from build123d import *

# Parameters (mm, degrees)
SKETCH1_R           = 10
SKETCH1_R_2         = 1.65
BOSS_EXTRUDE1_DEPTH = 2
SKETCH2_R           = 16
BOSS_EXTRUDE2_DEPTH = 8
BOSS_EXTRUDE3_DEPTH = 12
SKETCH4_R           = 1.65
CUT_EXTRUDE1_DEPTH  = 12
SKETCH5_R           = 2.8
CUT_EXTRUDE2_DEPTH  = 5.6


with BuildPart() as part:
    # Sketch1 → Boss-Extrude1 (new body)
    with BuildSketch(Plane.XY):
        Circle(SKETCH1_R)
        with Locations((0, 7)):
            Circle(SKETCH1_R_2, mode=Mode.SUBTRACT)
        with Locations((7, 0)):
            Circle(SKETCH1_R_2, mode=Mode.SUBTRACT)
        with Locations((0, -7)):
            Circle(SKETCH1_R_2, mode=Mode.SUBTRACT)
        with Locations((-7, 0)):
            Circle(SKETCH1_R_2, mode=Mode.SUBTRACT)
    extrude(amount=BOSS_EXTRUDE1_DEPTH)

    # Sketch2 → Boss-Extrude2 (add)
    with BuildSketch(Plane.XY.offset(2)):
        Circle(SKETCH2_R)
    extrude(amount=BOSS_EXTRUDE2_DEPTH)

    # Sketch3 → Boss-Extrude3 (add)
    with BuildSketch(Plane.XY.offset(10)):
        Polygon((3.868246804, 0), (1.934123402, 3.35), (-1.934123402, 3.35), (-3.868246804, 0), (-1.934123402, -3.35), (1.934123402, -3.35), align=None)
    extrude(amount=BOSS_EXTRUDE3_DEPTH)

    # Sketch4 → Cut-Extrude1 (cut)
    with BuildSketch(Plane(origin=(0, 0, 0), x_dir=(-1, 0, 0), z_dir=(0, 0, -1))):
        with Locations(Location((0, -7, 0), (0, 0, 180))):
            Circle(SKETCH4_R)
        with Locations(Location((-7, 0, 0), (0, 0, 180))):
            Circle(SKETCH4_R)
        with Locations(Location((7, 0, 0), (0, 0, 180))):
            Circle(SKETCH4_R)
        with Locations(Location((0, 7, 0), (0, 0, 180))):
            Circle(SKETCH4_R)
    extrude(amount=-CUT_EXTRUDE1_DEPTH, mode=Mode.SUBTRACT)

    # Sketch5 → Cut-Extrude2 (cut)
    with BuildSketch(Plane.XY.offset(10)):
        with Locations((0, 7)):
            Circle(SKETCH5_R)
        with Locations((7, 0)):
            Circle(SKETCH5_R)
        with Locations((0, -7)):
            Circle(SKETCH5_R)
        with Locations((-7, 0)):
            Circle(SKETCH5_R)
    extrude(amount=-CUT_EXTRUDE2_DEPTH, mode=Mode.SUBTRACT)


solid = part.part
Check sheet for the modelled part. Datum: model origin and axes. Units: mm. A direction names the side the tool comes from. Round coordinates to 2 decimals unless told otherwise and drop trailing zeros. Write each loop counter-clockwise with the first axis right and the second up, starting at its lowest first coordinate (ties: lowest second). Pieces come first, ordered by that corner, then holes. Notation, with made-up numbers: (30.5, 16) - (78.5, 16) arc R20 ccw to (78.5, 49) - close; hole circle Ø2 at (84, -5.5). An arc over 180 degrees is marked (long way). Return JSON: item names as keys, results as strings.
Q1. Cross-section at D-D (z = 6). Record the boundary of the cut face in (x, y).
Returned:
{"outline": "circle Ø32 at (0, 0); hole circle Ø5.6 at (-7, 0); hole circle Ø5.6 at (0, -7); hole circle Ø5.6 at (0, 7); hole circle Ø5.6 at (7, 0)"}
Q2. Cross-section at B-B (y = -6). Record the boundary of the cut face in (x, z).
Returned:
{"outline": "(-14.83, 2) - (-8, 2) - (-8, 0) - (-1.31, 0) - (-1.31, 4.4) - (-2.62, 4.4) - (-2.62, 10) - (-14.83, 10) - close; (1.31, 0) - (8, 0) - (8, 2) - (14.83, 2) - (14.83, 10) - (2.62, 10) - (2.62, 4.4) - (1.31, 4.4) - close"}
Q3. Scan lines: L1, parallel to Y at x = 0, z = 2.1; L2, parallel to Y at x = 0, z = 8; L3, parallel to X at y = 2.5, z = 9.5. Record each from-to range of solid material in increasing order. Write a range as from..to.
Returned:
{"L1": "y = -16..-8.65, -5.35..5.35, 8.65..16", "L2": "y = -16..-9.8, -4.2..4.2, 9.8..16", "L3": "x = -15.8..-8.26, -5.74..5.74, 8.26..15.8"}
Q4. Access from +Z, -Z, +X, -X, +Y, -Y to the whole of each face (thin tool, end or side, straight path). Record for faces 4 (the cylindrical face through (-2.17, -9.76, 0.99)), 5 (the flat face through (0, 3.35, 16)), 6 (the cylindrical face through (-0.607, -9.733, 7.239)), 7 (the flat face through (-2.915, -1.652, 15.916)), 8 (the flat face through (2.888, -1.698, 15.916)).
Returned:
{"face 4": "-Z", "face 5": "+Z, +X, -X, +Y", "face 6": "+Z", "face 7": "+Z, -X, -Y", "face 8": "+Z, +X, -Y"}
Q5. Depth check by flat-ended pin: P1, Ø5, axis at x = 0.5, z = 17, coming from the +Y side; P2, Ø2, axis at x = -7, y = 9, coming from the -Z side; P3, Ø6, axis at x = -11, z = 9, coming from the -Y side. Enter the tip coordinate at first touch or a pass-through.
Returned:
{"P1": "stops at y = 3.35", "P2": "stops at z = 2", "P3": "stops at y = -13.86"}
Q6. Cross-section at C-C (x = -7). Record the boundary of the cut face in (y, z).
Returned:
{"outline": "(-14.39, 2) - (-7.14, 2) - (-7.14, 0) - (-1.65, 0) - (-1.65, 4.4) - (-2.8, 4.4) - (-2.8, 10) - (-14.39, 10) - close; (1.65, 0) - (7.14, 0) - (7.14, 2) - (14.39, 2) - (14.39, 10) - (2.8, 10) - (2.8, 4.4) - (1.65, 4.4) - close"}
Q7. Cross-section at A-A (x = 0). Record the boundary of the cut face in (y, z).
Returned:
{"outline": "(-16, 2) - (-10, 2) - (-10, 0) - (-8.65, 0) - (-8.65, 4.4) - (-9.8, 4.4) - (-9.8, 10) - (-16, 10) - close; (-5.35, 0) - (5.35, 0) - (5.35, 4.4) - (4.2, 4.4) - (4.2, 10) - (3.35, 10) - (3.35, 22) - (-3.35, 22) - (-3.35, 10) - (-4.2, 10) - (-4.2, 4.4) - (-5.35, 4.4) - close; (8.65, 0) - (10, 0) - (10, 2) - (16, 2) - (16, 10) - (9.8, 10) - (9.8, 4.4) - (8.65, 4.4) - close"}
Q8. Draft check along X on faces 1 (the cylindrical face through (-8.65, -0.07, 2.17)), 2 (the flat face through (10.4, 0.2, 2)), 3 (the cylindrical face through (-3.47, -15.62, 5.94)). Enter one of: released by +X, released by -X, zero draft, split by the parting line, or undercut.
Returned:
{"face 1": "undercut", "face 2": "zero draft", "face 3": "split by the parting line"}
